Geometry: final body of the model. Coordinates: model frame, mm. Face numbers are marked on the shaded views. A direction names the side the tool comes from. Give positions to 0.01 mm unless a question says otherwise; leave off trailing zeros. Write each loop counter-clockwise with the first axis right and the second up, starting at its lowest first coordinate (ties: lowest second). Pieces come first, ordered by that corner, then holes.
Q1. Cut plane B-B on z = -4. Return the cut outline in (x, y), plus the area to 3 significant figures.
Q2. Line query: L1, parallel to Z at x = 24, y = 6; L2, parallel to X at y = 1, z = -13.75; L3, parallel to Z at x = 13.75, y = 5.5. Output: solid intervals per line, ascending.
Q3. Cut plane D-D on z = -14. Return the cut outline in (x, y), plus the area to 3 significant figures.
Q4. Draft query along X for the marked faces 3, 4, 5 and 6. Return one class per face: pulls with the +X half, pulls with the -X half, needs draft (parallel to the pull), parting line crosses it, or undercut.
Q5. Reachability of the marked faces 1 and 2 from +Z, -Z, +X, -X, +Y, -Y: full face, straight path, thin tool, end or side. Return the list, or none.
Q6. Cut plane A-A on x = 4. Return the cut outline in (y, z).
Q7. Cut plane C-C on x = 14. Return the cut outline in (y, z), plus the area to 3 significant figures.
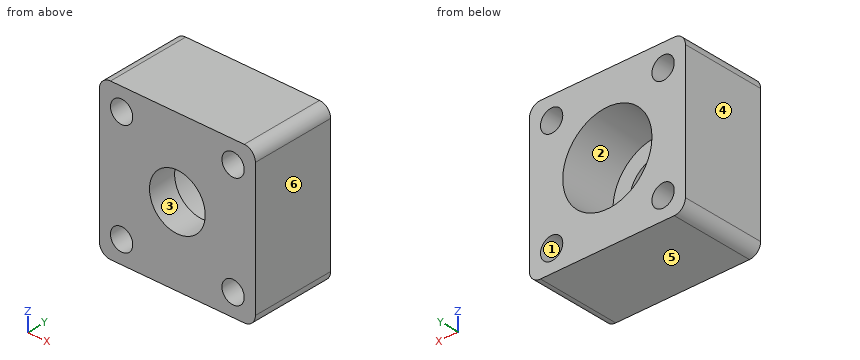
```python
from build123d import *

# Parameters (mm, degrees)
SKETCH1_W           = 28
SKETCH1_H           = 28
BOSS_EXTRUDE1_DEPTH = 15
SKETCH2_R           = 5
SKETCH2_R_2         = 2
CUT_EXTRUDE1_DEPTH  = 16
SKETCH3_R           = 8
CUT_EXTRUDE2_DEPTH  = 10
FILLET1_R           = 2


with BuildPart() as part:
    # Sketch1 → Boss-Extrude1 (new body)
    with BuildSketch(Plane(origin=(0, 0, 0), x_dir=(1, 0, 0), z_dir=(0, 1, 0))):
        with Locations((14, 14)):
            Rectangle(SKETCH1_W, SKETCH1_H)
    extrude(amount=BOSS_EXTRUDE1_DEPTH)

    # Sketch2 → Cut-Extrude1 (cut, through all)
    with BuildSketch(Plane(origin=(0, 15, 0), x_dir=(-1, 0, 0), z_dir=(0, 1, 0))):
        with Locations((-14, -14)):
            Circle(SKETCH2_R)
        with Locations((-4, -24)):
            Circle(SKETCH2_R_2)
        with Locations((-24, -24)):
            Circle(SKETCH2_R_2)
        with Locations((-4, -4)):
            Circle(SKETCH2_R_2)
        with Locations((-24, -4)):
            Circle(SKETCH2_R_2)
    extrude(amount=-CUT_EXTRUDE1_DEPTH, mode=Mode.SUBTRACT)

    # Sketch3 → Cut-Extrude2 (cut)
    with BuildSketch(Plane(origin=(0, 15, 0), x_dir=(1, 0, 0), z_dir=(0, 1, 0))):
        with Locations((14, 14)):
            Circle(SKETCH3_R)
    extrude(amount=-CUT_EXTRUDE2_DEPTH, mode=Mode.SUBTRACT)

    # Fillet1
    fillet1_edges = [part.edges().sort_by_distance(p)[0] for p in [
        (0, 7.5, 0),
        (0, 7.5, -28),
        (28, 7.5, -28),
        (28, 7.5, 0),
    ]]
    fillet(fillet1_edges, radius=FILLET1_R)


solid = part.part
```
Data:
1. outline: (0, 0) - (2, 0) - (2, 15) - (0, 15) - close; (6, 0) - (22, 0) - (22, 15) - (6, 15) - close; (26, 0) - (28, 0) - (28, 15) - (26, 15) - close
1. area: 300 mm2
2. L1: z = -28 to -26, -22 to -6, -2 to 0
2. L2: x = 0 to 9.01, 18.99 to 28
2. L3: z = -28 to -22, -6 to 0
3. outline: (0, 0) - (9, 0) - (9, 5) - (6, 5) - (6, 15) - (0, 15) - close; (19, 0) - (28, 0) - (28, 15) - (22, 15) - (22, 5) - (19, 5) - close
3. area: 210 mm2
4. face 3: undercut
4. face 4: pulls with the -X half
4. face 5: needs draft
4. face 6: pulls with the +X half
5. face 1: +Y, -Y
5. face 2: +Y
6. outline: (0, -28) - (15, -28) - (15, -26) - (0, -26) - close; (0, -22) - (15, -22) - (15, -6) - (0, -6) - close; (0, -2) - (15, -2) - (15, 0) - (0, 0) - close
7. outline: (0, -28) - (15, -28) - (15, -22) - (5, -22) - (5, -19) - (0, -19) - close; (0, -9) - (5, -9) - (5, -6) - (15, -6) - (15, 0) - (0, 0) - close
7. area: 210 mm2
